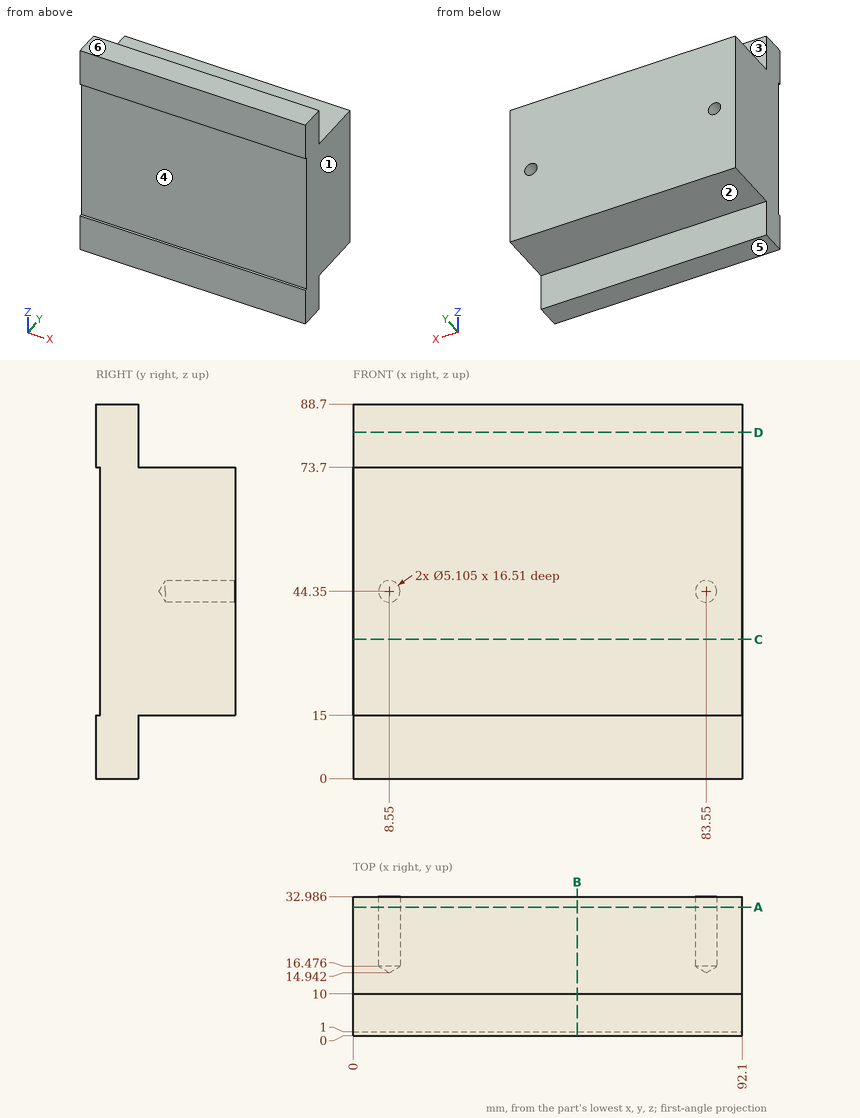
Source: three-view drawing plus pictorial views. Frame: mm from the lowest corner of the part. A direction names the side the tool comes from. Give positions to 0.01 mm unless a question says otherwise; leave off trailing zeros. Write each loop counter-clockwise with the first axis right and the second up, starting at its lowest first coordinate (ties: lowest second). Pieces come first, ordered by that corner, then holes. Notation, with made-up numbers: (-9.75, 53) -> (31.25, 53) arc R22 ccw to (31.25, 89) -> close; hole circle Ø2 at (70, 76). An arc over 180 degrees is marked (long way). Write item = value, one per line.
Q1. Cut plane D-D on z = 82. Return loops of the section in (x, y).
Here are the results:
outline = (0, 0) -> (92.1, 0) -> (92.1, 10) -> (0, 10) -> close
Q2. Cut plane B-B on x = 53. Return loops of the section in (y, z), then the cut area to 3 significant figures.
Here are the results:
outline = (0, 0) -> (10, 0) -> (10, 15) -> (32.99, 15) -> (32.99, 73.7) -> (10, 73.7) -> (10, 88.7) -> (0, 88.7) -> (0, 73.7) -> (1, 73.7) -> (1, 15) -> (0, 15) -> close
area = 2,180 mm²
Q3. Line query: line 1 (X direction, y = 28, z = 44.35); line 2 (Z direction, x = 8.55, y = 27); line 3 (Y direction, x = 39.5, z = 9). Output: solid intervals per line, ascending. Write a range as from..to.
Here are the results:
line_1 = 0..6, 11.1..81, 86.1..92.1
line_2 = 15..41.8, 46.9..73.7
line_3 = 0..10
Q4. First-contact query: pin 1 (4 mm diameter, centred on y = 10, z = 30, fed in from -X); pin 2 (4 mm diameter, centred on x = 83.55, z = 44.35, fed in from +Y) (1 decimal); pin 3 (4 mm diameter, centred on x = 25, z = 36, fed in from -Y); pin 4 (16.5 mm diameter, centred on x = 42, z = 5, fed in from +Y). Flat tips, straight axial feed; report the tip coordinate or a pass-through.
Here are the results:
pin_1 = 0
pin_2 = 16.1
pin_3 = 1
pin_4 = 10
Q5. Reachability of the marked faces 1, 2 and 3 from +Z, -Z, +X, -X, +Y, -Y: full face, straight path, thin tool, end or side. Return the list, or none.
Here are the results:
face_1 = +Z, -Z, +X, +Y, -Y
face_2 = -Z, +X, -X, +Y
face_3 = +Z, +X, -X, +Y
Q6. Cut plane C-C on z = 33. Return loops of the section in (x, y), then the cut area to 3 significant figures.
Here are the results:
outline = (0, 1) -> (92.1, 1) -> (92.1, 32.99) -> (0, 32.99) -> close
area = 2,950 mm²
Q7. Mould query, pull axis Z, two halves, no side actions, for the marked faces 4, 5 and 6. Classes: +Z half, -Z half, draft (parallel to the pull), parting line (faces both ways), or undercut.
Here are the results:
face_4 = undercut
face_5 = -Z half
face_6 = +Z half
Q8. Cut plane A-A on y = 30.5. State how many separate pieces and enclosed holes the cut face has, then the cut area to 3 significant figures.
Here are the results:
separate_pieces = 1
enclosed_holes = 2
area = 5,370 mm²
